Geometry check sheet. Reference: the model listing, model coordinates, mm. Give positions to 0.01 mm unless a question says otherwise; leave off trailing zeros. Loops run counter-clockwise (first coordinate to the right, second up) from the corner with the lowest first, then second, coordinate; pieces in that order, holes last. Notation, with made-up numbers: (-2, 88.5) -> (37, 88.5) arc R20 ccw to (37, 112.5) -> close; hole circle Ø3 at (45, 32.25). An arc over 180 degrees is marked (long way). One line per question, with ' | ' between items.
from build123d import *

# Parameters (mm, degrees)
SKETCH1_W           = 112.7
SKETCH1_H           = 112.7
BOSS_EXTRUDE1_DEPTH = 6.35
SKETCH2_W           = 12.7
SKETCH2_H           = 6.35
CUT_EXTRUDE2_DEPTH  = 7.35
CIRPATTERN1_COUNT   = 4
SKETCH5_W           = 6.35
SKETCH5_H           = 19.05
CUT_EXTRUDE3_DEPTH  = 7.35
SKETCH6_W           = 12.7
SKETCH6_H           = 6.35
CUT_EXTRUDE4_DEPTH  = 7.35
CIRPATTERN2_COUNT   = 4
CIRPATTERN3_COUNT   = 4
SKETCH7_W           = 40
SKETCH7_H           = 40
CUT_EXTRUDE5_DEPTH  = 7.35
CUT_EXTRUDE6_START  = -7.35
CUT_EXTRUDE6_DEPTH  = 8.35


with BuildPart() as part:
    # Sketch1 → Boss-Extrude1 (new body)
    with BuildSketch(Plane(origin=(0, 0, 0), x_dir=(1, 0, 0), z_dir=(0, 1, 0))):
        Rectangle(SKETCH1_W, SKETCH1_H)
    extrude(amount=BOSS_EXTRUDE1_DEPTH)

    # Sketch2 → Cut-Extrude2 (cut, through all)
    with BuildSketch(Plane(origin=(0, 6.35, 0), x_dir=(1, 0, 0), z_dir=(0, 1, 0))):
        with Locations((0, 53.175)):
            Rectangle(SKETCH2_W, SKETCH2_H)
    cut_extrude2 = extrude(amount=-CUT_EXTRUDE2_DEPTH, mode=Mode.SUBTRACT)

    # CirPattern1: Cut-Extrude2 ×4 about axis
    cirpattern1_axis = Axis((0, 0, 0), (0, 1, 0))
    for i in range(1, CIRPATTERN1_COUNT):
        add(cut_extrude2.rotate(cirpattern1_axis, i * 360 / CIRPATTERN1_COUNT), mode=Mode.SUBTRACT)

    # Sketch5 → Cut-Extrude3 (cut, through all)
    with BuildSketch(Plane(origin=(0, 6.35, 0), x_dir=(1, 0, 0), z_dir=(0, 1, 0))):
        with Locations((53.175, -46.825)):
            Rectangle(SKETCH5_W, SKETCH5_H)
    cut_extrude3 = extrude(amount=-CUT_EXTRUDE3_DEPTH, mode=Mode.SUBTRACT)

    # Sketch6 → Cut-Extrude4 (cut, through all)
    with BuildSketch(Plane(origin=(0, 6.35, 0), x_dir=(1, 0, 0), z_dir=(0, 1, 0))):
        with Locations((43.65, -53.175)):
            Rectangle(SKETCH6_W, SKETCH6_H)
    cut_extrude4 = extrude(amount=-CUT_EXTRUDE4_DEPTH, mode=Mode.SUBTRACT)

    # CirPattern2: Cut-Extrude3 ×4 about axis
    cirpattern2_axis = Axis((0, 0, 0), (0, 1, 0))
    for i in range(1, CIRPATTERN2_COUNT):
        add(cut_extrude3.rotate(cirpattern2_axis, i * 360 / CIRPATTERN2_COUNT), mode=Mode.SUBTRACT)

    # CirPattern3: Cut-Extrude4 ×4 about axis
    cirpattern3_axis = Axis((0, 0, 0), (0, 1, 0))
    for i in range(1, CIRPATTERN3_COUNT):
        add(cut_extrude4.rotate(cirpattern3_axis, i * 360 / CIRPATTERN3_COUNT), mode=Mode.SUBTRACT)

    # Sketch7 → Cut-Extrude5 (cut, through all)
    with BuildSketch(Plane(origin=(0, 6.35, 0), x_dir=(1, 0, 0), z_dir=(0, 1, 0))):
        with Locations((20, -20)):
            Rectangle(SKETCH7_W, SKETCH7_H)
    extrude(amount=-CUT_EXTRUDE5_DEPTH, mode=Mode.SUBTRACT)

    # Sketch8 → Cut-Extrude6 (cut)
    with BuildSketch(Plane(origin=(0, 6.35, 0), x_dir=(1, 0, 0), z_dir=(0, 1, 0)).offset(CUT_EXTRUDE6_START)):
        with BuildLine():
            Line((40, -35), (40, -40))
            ThreePointArc((40, -40), (42.5, -37.5), (40, -35))
        make_face()
    cut_extrude6 = extrude(amount=CUT_EXTRUDE6_DEPTH, mode=Mode.SUBTRACT)

    # Mirror1: Cut-Extrude6 across plane
    add(cut_extrude6.mirror(Plane(origin=(0, 3.175, 20), x_dir=(1, 0, 0), z_dir=(0, 0, 1))), mode=Mode.SUBTRACT)


solid = part.part
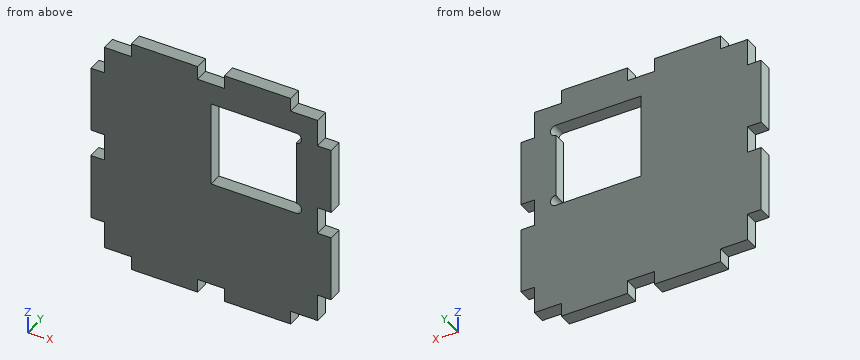
Item 1: Depth check by flat-ended pin: pin 1 Ø5 at (x, z) = (25, -35.5) entering from -Y; pin 2 Ø3 at (x, y) = (52.5, 4.5) entering from +Z; pin 3 Ø3 at (y, z) = (2, -53) entering from -X; pin 4 Ø1.9 at (x, y) = (54, 4) entering from -Z. Enter the tip coordinate at first touch or a pass-through.
Result:
pin 1: y = 0 | pin 2: z = 37.3 | pin 3: x = -37.3 | pin 4: z = -37.3
Item 2: Scan lines: probe 1 along Z at (x, y) = (15, 1); probe 2 along X at (y, z) = (1, -38). Record each from-to range of solid material in increasing order.
Result:
probe 1: -56.35 to 0, 40 to 56.35 | probe 2: -50 to 50
Item 3: Sectioned sample at B-B (z = 44.5). Record the cut outline in (x, y).
Result:
outline: (-50, 0) -> (50, 0) -> (50, 6.35) -> (-50, 6.35) -> close
Item 4: Sectioned sample at A-A (z = 2.5). Record the cut outline in (x, y).
Result:
outline: (-50, 0) -> (0, 0) -> (0, 6.35) -> (-50, 6.35) -> close; (42.5, 0) -> (50, 0) -> (50, 6.35) -> (42.5, 6.35) -> close
